Here's how the part is built. I have some questions about the finished solid (model axes, mm). Face numbers are marked on the shaded views. A direction names the side the tool comes from. Round coordinates to 2 decimals unless told otherwise and drop trailing zeros. Loops run counter-clockwise (first coordinate to the right, second up) from the corner with the lowest first, then second, coordinate; pieces in that order, holes last. Notation, with made-up numbers: M -0.5,-21 L 12.5,-21 A33 cw 12.5,9 Z; hole C 2,-23 d9. An arc over 180 degrees is marked long. Answer as a JSON object with one key per item and string values.
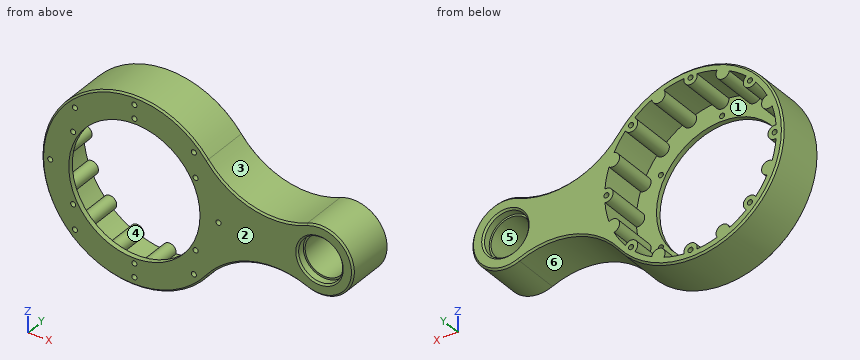
from build123d import *

# Parameters (mm, degrees)
SKETCH1_R           = 55
SKETCH1_R_2         = 39
SKETCH1_R_3         = 1.5
BOSS_EXTRUDE1_DEPTH = 3
SKETCH2_R           = 55
SKETCH2_R_2         = 1.5
BOSS_EXTRUDE3_DEPTH = 27
BOSS_EXTRUDE4_START = -30
SKETCH3_R           = 13.1
BOSS_EXTRUDE4_DEPTH = 30
BOSS_EXTRUDE5_START = -5
SKETCH6_R           = 13.1
SKETCH6_R_2         = 12
BOSS_EXTRUDE5_DEPTH = 20
CHAMFER1_SIZE       = 1


with BuildPart() as part:
    # Sketch1 → Boss-Extrude1 (new body)
    with BuildSketch(Plane(origin=(0, 0, 0), x_dir=(1, 0, 0), z_dir=(0, 1, 0))):
        Circle(SKETCH1_R)
        Circle(SKETCH1_R_2, mode=Mode.SUBTRACT)
        with Locations((0, 50)):
            Circle(SKETCH1_R_3, mode=Mode.SUBTRACT)
        with Locations((35.355339059, 35.355339059)):
            Circle(SKETCH1_R_3, mode=Mode.SUBTRACT)
        with Locations((50, 0)):
            Circle(SKETCH1_R_3, mode=Mode.SUBTRACT)
        with Locations((35.355339059, -35.355339059)):
            Circle(SKETCH1_R_3, mode=Mode.SUBTRACT)
        with Locations((0, -50)):
            Circle(SKETCH1_R_3, mode=Mode.SUBTRACT)
        with Locations((-35.355339059, -35.355339059)):
            Circle(SKETCH1_R_3, mode=Mode.SUBTRACT)
        with Locations((-50, 0)):
            Circle(SKETCH1_R_3, mode=Mode.SUBTRACT)
        with Locations((-35.355339059, 35.355339059)):
            Circle(SKETCH1_R_3, mode=Mode.SUBTRACT)
        with Locations((0, 42)):
            Circle(SKETCH1_R_3, mode=Mode.SUBTRACT)
        with Locations((36.373066959, 21)):
            Circle(SKETCH1_R_3, mode=Mode.SUBTRACT)
        with Locations((36.373066959, -21)):
            Circle(SKETCH1_R_3, mode=Mode.SUBTRACT)
        with Locations((0, -42)):
            Circle(SKETCH1_R_3, mode=Mode.SUBTRACT)
        with Locations((-36.373066959, -21)):
            Circle(SKETCH1_R_3, mode=Mode.SUBTRACT)
        with Locations((-36.373066959, 21)):
            Circle(SKETCH1_R_3, mode=Mode.SUBTRACT)
    extrude(amount=BOSS_EXTRUDE1_DEPTH)

    # Sketch2 → Boss-Extrude3 (add)
    with BuildSketch(Plane(origin=(0, 3, 0), x_dir=(1, 0, 0), z_dir=(0, 1, 0))):
        Circle(SKETCH2_R)
        with Locations((-35.355339059, 35.355339059)):
            Circle(SKETCH2_R_2, mode=Mode.SUBTRACT)
        with Locations((-50, 0)):
            Circle(SKETCH2_R_2, mode=Mode.SUBTRACT)
        with Locations((-35.355339059, -35.355339059)):
            Circle(SKETCH2_R_2, mode=Mode.SUBTRACT)
        with Locations((0, -50)):
            Circle(SKETCH2_R_2, mode=Mode.SUBTRACT)
        with Locations((35.355339059, -35.355339059)):
            Circle(SKETCH2_R_2, mode=Mode.SUBTRACT)
        with Locations((50, 0)):
            Circle(SKETCH2_R_2, mode=Mode.SUBTRACT)
        with Locations((35.355339059, 35.355339059)):
            Circle(SKETCH2_R_2, mode=Mode.SUBTRACT)
        with Locations((0, 50)):
            Circle(SKETCH2_R_2, mode=Mode.SUBTRACT)
        with BuildLine():
            ThreePointArc((-3.908644266, 50.85), (0, 46), (3.908644266, 50.85))
            ThreePointArc((3.908644266, 50.85), (9.949606423, 50.020049301), (15.848336098, 48.475047632))
            ThreePointArc((15.848336098, 48.475047632), (17.603437889, 42.498458496), (23.070568973, 45.483500825))
            ThreePointArc((23.070568973, 45.483500825), (28.334081884, 42.404950227), (33.192550957, 38.720208689))
            ThreePointArc((33.192550957, 38.720208689), (32.526911935, 32.526911935), (38.720208689, 33.192550957))
            ThreePointArc((38.720208689, 33.192550957), (42.404950227, 28.334081884), (45.483500825, 23.070568973))
            ThreePointArc((45.483500825, 23.070568973), (42.498458496, 17.603437889), (48.475047632, 15.848336098))
            ThreePointArc((48.475047632, 15.848336098), (50.020049301, 9.949606423), (50.85, 3.908644266))
            ThreePointArc((50.85, 3.908644266), (46, 0), (50.85, -3.908644266))
            ThreePointArc((50.85, -3.908644266), (50.020049301, -9.949606423), (48.475047632, -15.848336098))
            ThreePointArc((48.475047632, -15.848336098), (42.498458496, -17.603437889), (45.483500825, -23.070568973))
            ThreePointArc((45.483500825, -23.070568973), (42.404950227, -28.334081884), (38.720208689, -33.192550957))
            ThreePointArc((38.720208689, -33.192550957), (32.526911935, -32.526911935), (33.192550957, -38.720208689))
            ThreePointArc((33.192550957, -38.720208689), (28.334081884, -42.404950227), (23.070568973, -45.483500825))
            ThreePointArc((23.070568973, -45.483500825), (17.603437889, -42.498458496), (15.848336098, -48.475047632))
            ThreePointArc((15.848336098, -48.475047632), (9.949606423, -50.020049301), (3.908644266, -50.85))
            ThreePointArc((3.908644266, -50.85), (0, -46), (-3.908644266, -50.85))
            ThreePointArc((-3.908644266, -50.85), (-9.949606423, -50.020049301), (-15.848336098, -48.475047632))
            ThreePointArc((-15.848336098, -48.475047632), (-17.603437889, -42.498458496), (-23.070568973, -45.483500825))
            ThreePointArc((-23.070568973, -45.483500825), (-28.334081884, -42.404950227), (-33.192550957, -38.720208689))
            ThreePointArc((-33.192550957, -38.720208689), (-32.526911935, -32.526911935), (-38.720208689, -33.192550957))
            ThreePointArc((-38.720208689, -33.192550957), (-42.404950227, -28.334081884), (-45.483500825, -23.070568973))
            ThreePointArc((-45.483500825, -23.070568973), (-42.498458496, -17.603437889), (-48.475047632, -15.848336098))
            ThreePointArc((-48.475047632, -15.848336098), (-50.020049301, -9.949606423), (-50.85, -3.908644266))
            ThreePointArc((-50.85, -3.908644266), (-46, 0), (-50.85, 3.908644266))
            ThreePointArc((-50.85, 3.908644266), (-50.020049301, 9.949606423), (-48.475047632, 15.848336098))
            ThreePointArc((-48.475047632, 15.848336098), (-42.498458496, 17.603437889), (-45.483500825, 23.070568973))
            ThreePointArc((-45.483500825, 23.070568973), (-42.404950227, 28.334081884), (-38.720208689, 33.192550957))
            ThreePointArc((-38.720208689, 33.192550957), (-32.526911935, 32.526911935), (-33.192550957, 38.720208689))
            ThreePointArc((-33.192550957, 38.720208689), (-28.334081884, 42.404950227), (-23.070568973, 45.483500825))
            ThreePointArc((-23.070568973, 45.483500825), (-17.603437889, 42.498458496), (-15.848336098, 48.475047632))
            ThreePointArc((-15.848336098, 48.475047632), (-9.949606423, 50.020049301), (-3.908644266, 50.85))
        make_face(mode=Mode.SUBTRACT)
    extrude(amount=BOSS_EXTRUDE3_DEPTH)

    # Sketch3 → Boss-Extrude4 (add)
    with BuildSketch(Plane(origin=(0, 30, 0), x_dir=(1, 0, 0), z_dir=(0, 1, 0)).offset(BOSS_EXTRUDE4_START)):
        with BuildLine():
            ThreePointArc((43.392857143, -33.794377476), (55, 0), (43.392857143, 33.794377476))
            ThreePointArc((43.392857143, 33.794377476), (70.212437062, 16.137600278), (102.24025974, 18.433296805))
            ThreePointArc((102.24025974, 18.433296805), (130, 0), (102.24025974, -18.433296805))
            ThreePointArc((102.24025974, -18.433296805), (70.212437062, -16.137600278), (43.392857143, -33.794377476))
        make_face()
        with Locations((110, 0)):
            Circle(SKETCH3_R, mode=Mode.SUBTRACT)
    extrude(amount=BOSS_EXTRUDE4_DEPTH)

    # Sketch6 → Boss-Extrude5 (add)
    with BuildSketch(Plane(origin=(0, 30, 0), x_dir=(1, 0, 0), z_dir=(0, 1, 0)).offset(BOSS_EXTRUDE5_START)):
        with Locations((110, 0)):
            Circle(SKETCH6_R)
        with Locations((110, 0)):
            Circle(SKETCH6_R_2, mode=Mode.SUBTRACT)
    extrude(amount=-BOSS_EXTRUDE5_DEPTH)

    # Chamfer1
    chamfer1_edges = [part.edges().sort_by_distance(p)[0] for p in [
        (-55, 30, 0),
        (-55, 0, 0),
        (130, 30, 0),
        (70.212437062, 0, -16.137600278),
        (70.212437062, 0, 16.137600278),
        (96.9, 0, 0),
        (70.212437062, 30, -16.137600278),
        (70.212437062, 30, 16.137600278),
        (130, 0, 0),
        (96.9, 30, 0),
    ]]
    chamfer(chamfer1_edges, length=CHAMFER1_SIZE)


solid = part.part
Item 1: I'm going to push flat-ended pins straight in: pin 1 Ø1 at (y, z) = (19.5, -28) entering from -X; pin 2 Ø3 at (x, y) = (-33, 3) entering from +Z; pin 3 Ø4 at (x, z) = (-35.36, 35.36) entering from -Y; pin 4 Ø6 at (y, z) = (4, 10.5) entering from +X. Where does each tip first touch, or does it pass through?
Resolved:
{"pin 1": "x = -47.63", "pin 2": "z = 45.09", "pin 3": "y = 0", "pin 4": "x = 128.54"}
Item 2: Please list where these lines run through material, in increasing order: probe 1 along Z at (x, y) = (0, 18); probe 2 along Z at (x, y) = (48, 25); probe 3 along X at (y, z) = (26.5, 44). Write a range as from..to.
Resolved:
{"probe 1": "-55..-51.5, -48.5..-46, 46..48.5, 51.5..55", "probe 2": "-28.65..-15.57, -3.46..3.46, 15.57..28.65", "probe 3": "-33..-25.79, -22.48..-15.79, 15.79..22.48, 25.79..33"}
Item 3: On a 3-axis mill with a long thin cutter (end or side, diameter ignored), from which of +Z, -Z, +X, -X, +Y, -Y can I reach the whole of each face in a straight line? I mean the marked faces 1 and 2. Say none if no direction works.
Resolved:
{"face 1": "+Y", "face 2": "+Z, -Z, +X, -X, -Y"}
Item 4: If we mould it in two halves opening along Z, with no side actions, what happens to the marked faces 3, 4, 5 and 6? For each: pulls with the +Z half, pulls with the -Z half, needs draft (parallel to the pull), parting line crosses it, or undercut.
Resolved:
{"face 3": "pulls with the +Z half", "face 4": "undercut", "face 5": "undercut", "face 6": "pulls with the -Z half"}
Item 5: I want a section at B-B, the plane y = 8.25. State how many separate pieces and enclosed holes the cut face has, then the cut area to 3 significant figures.
Resolved:
{"separate pieces": "1", "enclosed holes": "10", "area": "3,960 mm²"}
Item 6: I want a section at A-A, the plane x = 110. Please give me the cut outline in (y, z).
Resolved:
{"outline": "M 0,-19 L 1,-20 L 29,-20 L 30,-19 L 30,-14.1 L 29,-13.1 L 25,-13.1 L 25,-12 L 5,-12 L 5,-13.1 L 1,-13.1 L 0,-14.1 Z; M 0,14.1 L 1,13.1 L 5,13.1 L 5,12 L 25,12 L 25,13.1 L 29,13.1 L 30,14.1 L 30,19 L 29,20 L 1,20 L 0,19 Z"}
